```python
from build123d import *

# Parameters (mm, degrees)
F0_W     = 100
F0_H     = 80
F1_DEPTH = 20
F2_W     = 60
F2_H     = 40
F3_DEPTH = 50
F5_DEPTH = 81


with BuildPart() as f1:
    # F0 (on Top) → F1 (new body)
    with BuildSketch(Plane.XY):
        Rectangle(F0_W, F0_H)
    extrude(amount=F1_DEPTH)

    # F2 (on face) → F3 (join)
    with BuildSketch(Plane.XY.offset(20)):
        Rectangle(F2_W, F2_H)
    extrude(amount=F3_DEPTH)

    # F4 (on face) → F5 (cut)
    with BuildSketch(Plane(origin=(-30, 0, 0), x_dir=(0, -1, 0), z_dir=(-1, 0, 0))):
        Polygon((10, 70), (-10, 70), (0, 60), align=None)
    extrude(amount=-F5_DEPTH, mode=Mode.SUBTRACT)


solid = f1.part
```
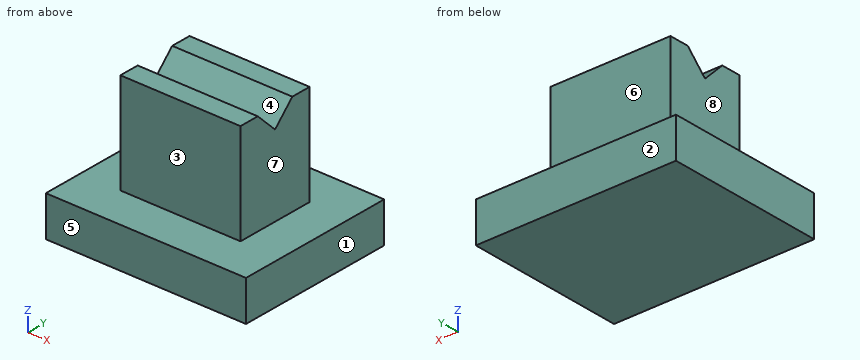
Could you check a few things on this model? Use its own coordinates, in mm. Face numbers are marked on the shaded views. A direction names the side the tool comes from. Give positions to 0.01 mm unless a question says otherwise; leave off trailing zeros. Order: outer loops, then holes, each group sorted by start corner. A loop starts at its lowest first (then second) coordinate and runs counter-clockwise, first axis right, second up.
Q1. Suppose I cut it at C-C, the plane z = 36. Write out the boundary of the cut face in (x, y).
Q2. Suppose I cut it at D-D, the plane x = -43. Write out the boundary of the cut face in (y, z), and give its area (3 significant figures).
Q3. We'd pull the mould along Y, two halves only. Please class the marked faces 1, 2, 3 and 4: +Y half, -Y half, draft (parallel to the pull), parting line (faces both ways), or undercut.
Q4. Suppose I cut it at B-B, the plane x = -3. Write out the boundary of the cut face in (y, z).
Q5. If I drill on line 1 along Y through (x, z) = (22.5, 57); line 2 along Z through (x, y) = (4.5, -21); line 3 along X through (y, z) = (-11.5, 29.5), over which ranges is the centre line in solid material (lowest first)?
Q6. Suppose I cut it at A-A, the plane y = 8. Write out the boundary of the cut face in (x, z), and give its area (3 significant figures).
Q7. I'm going to push flat-ended pins straight in: P1, Ø20, axis at y = -4, z = 46.5, coming from the +X side; P2, Ø5, axis at y = -22, z = 38, coming from the -X side; P3, Ø5, axis at x = -24.5, y = -24.5, coming from the -Z side; P4, Ø6, axis at x = -22.5, y = -3.5, coming from the +Z side. Where does each tip first touch, or does it pass through?
Q8. For the marked faces 5, 6, 7 and 8, which set-ups out of +Z, -Z, +X, -X, +Y, -Y let a thin tool reach every point of the face, with its end or its side?
Solution:
1. outline: (-30, -20) - (30, -20) - (30, 20) - (-30, 20) - close
2. outline: (-40, 0) - (40, 0) - (40, 20) - (-40, 20) - close
2. area: 1,600 mm2
3. face 1: draft
3. face 2: +Y half
3. face 3: -Y half
3. face 4: undercut
4. outline: (-40, 0) - (40, 0) - (40, 20) - (20, 20) - (20, 70) - (10, 70) - (0, 60) - (-10, 70) - (-20, 70) - (-20, 20) - (-40, 20) - close
5. line 1: y = -20 to 20
5. line 2: z = 0 to 20
5. line 3: x = -30 to 30
6. outline: (-50, 0) - (50, 0) - (50, 20) - (30, 20) - (30, 68) - (-30, 68) - (-30, 20) - (-50, 20) - close
6. area: 4,880 mm2
7. P1: stops at x = 30
7. P2: stops at x = -30
7. P3: stops at z = 0
7. P4: stops at z = 66.5
8. face 5: +Z, -Z, +X, -X, -Y
8. face 6: +Z, +X, -X, +Y
8. face 7: +Z, +X, +Y, -Y
8. face 8: +Z, -X, +Y, -Y
